For this review, take the finished solid that the model builds, in its own axes (mm). A direction names the side the tool comes from. Round coordinates to 2 decimals unless told otherwise and drop trailing zeros. Loops run counter-clockwise (first coordinate to the right, second up) from the corner with the lowest first, then second, coordinate; pieces in that order, holes last.
1. Clearance check with flat-ended pins moving along their axes: pin 1 Ø7.5 at (x, z) = (0, 0) entering from +Y; pin 2 Ø1 at (y, z) = (-1, 0.5) entering from +X; pin 3 Ø0.9 at (y, z) = (-1.5, 5.5) entering from +X; pin 4 Ø1 at (x, y) = (10, -3.5) entering from +Z. State where each tip first meets the part, or that it passes through.
2. Consider section C-C on x = 5.75. State the section outline as (y, z) points.
3. Draft analysis for pull direction X (two halves, no side actions). For faces 4 (the flat face through (0, -4.737, -6)), 5 (the flat face through (-12.131, -2.335, 4.043)), 6 (the flat face through (10.671, -2.335, -7.045)), 7 (the flat face through (12.527, -2.335, 2.564)), state which applies: released by +X, released by -X, zero draft, split by the parting line, or undercut.
4. Consider section D-D on x = -8. State the section outline as (y, z) points.
5. Consider section B-B on x = 0. State the section outline as (y, z) points, then the cut area to 3 significant figures.
6. Tool access review of faces 1 (the flat face through (-8.484, -2.335, 9.567)), 2 (the flat face through (7.045, -2.335, 10.671)), 3 (the flat face through (11.66, -2.34, -1.53)): name each direction out of +Z, -Z, +X, -X, +Y, -Y from which nothing blocks a thin tool from reaching the whole face with its end or side.
7. Consider section A-A on z = 0. State the section outline as (x, y) points, then the cut area to 3 significant figures.
8. To check wall thickness, follow line 1 along Z through (x, y) = (12.25, -3.4); line 2 along X through (y, z) = (-1.4, 0); line 3 along Z through (x, y) = (0, -3.1). State the ranges of each line that lie inside material, in increasing order.
from build123d import *

# Parameters (mm, degrees)
F0_R            = 13.7922
F0_R_2          = 4.7752
F1_DEPTH        = 4.7371
F3_DEPTH        = 4.7381
F5_DEPTH        = 4.7381
F5_COPIES_COUNT = 24


# Not quite as in the source:
# - a pattern or mirror of a feature is missing from the dataset's text; its kind, count and spacing are read off the source's solid


with BuildPart() as f1:
    # F0 (on Front) → F1 (new body)
    with BuildSketch(Plane.XZ):
        Circle(F0_R)
        Circle(F0_R_2, mode=Mode.SUBTRACT)
    extrude(amount=F1_DEPTH)

    # F2 (on Front) → F3 (cut, through all)
    with BuildSketch(Plane.XZ):
        with BuildLine():
            Line((-1.5875, 6.3373), (-1.5875, 0))
            Line((-1.5875, 0), (1.5875, 0))
            Line((1.5875, 0), (1.5875, 6.3373))
            ThreePointArc((1.5875, 6.3373), (0, 7.9248), (-1.5875, 6.3373))
        make_face()
    extrude(amount=F3_DEPTH, mode=Mode.SUBTRACT)

    # F4 (on Front) → F5 (cut, through all)
    with BuildSketch(Plane.XZ):
        with BuildLine():
            Line((0.4064, 13.7922), (1.1320909341, 11.7126357032))
            Line((1.1320909341, 11.7126357032), (1.9379373174, 11.6065440142))
            Line((1.9379373174, 11.6065440142), (3.1771317781, 13.4274262413))
            ThreePointArc((3.1771317781, 13.4274262413), (1.8061892107, 13.7193691256), (0.4064, 13.7922))
        make_face()
    f5 = extrude(amount=F5_DEPTH, mode=Mode.SUBTRACT)

    # F5_copies: F5 ×24 about axis
    f5_copies_axis = Axis((0, 0, 0), (0, 1, 0))
    for i in range(1, F5_COPIES_COUNT):
        add(f5.rotate(f5_copies_axis, i * 360 / F5_COPIES_COUNT), mode=Mode.SUBTRACT)


solid = f1.part
Resolved:
1. pin 1: passes through
1. pin 2: stops at x = 13.79
1. pin 3: stops at x = 11.64
1. pin 4: stops at z = 10
2. outline: (-4.74, -11.46) - (0, -11.46) - (0, 11.46) - (-4.74, 11.46) - close
3. face 4: zero draft
3. face 5: released by -X
3. face 6: undercut
3. face 7: released by +X
4. outline: (-4.74, -9.33) - (0, -9.33) - (0, 9.33) - (-4.74, 9.33) - close
5. outline: (-4.74, -13.79) - (0, -13.79) - (0, -4.78) - (-4.74, -4.78) - close; (-4.74, 7.92) - (0, 7.92) - (0, 13.79) - (-4.74, 13.79) - close
5. area: 70.5 mm2
6. face 1: +Z, +Y, -Y
6. face 2: +Y, -Y
6. face 3: +X, +Y, -Y
7. outline: (-13.79, -4.74) - (-4.78, -4.74) - (-4.78, 0) - (-13.79, 0) - close; (4.78, -4.74) - (13.79, -4.74) - (13.79, 0) - (4.78, 0) - close
7. area: 85.4 mm2
8. line 1: z = -4.03 to -2.38, -0.94 to 0.94, 2.38 to 4.03
8. line 2: x = -13.79 to -4.78, 4.78 to 13.79
8. line 3: z = -13.79 to -4.78, 7.92 to 13.79
